from build123d import *

# Parameters (mm, degrees)
F0_W     = 8.3429142833
F0_H     = 111.0566146672
F1_DEPTH = 76.2
F0_W_2   = 108.8683158159
F0_H_2   = 0.4005401015
F2_DEPTH = 25.4
F3_SIZE  = 5.08
F4_DEPTH = 25.4


with BuildPart() as f1:
    # F0 (on Front) → F1 (new body)
    with BuildSketch(Plane.XZ):
        with Locations((-72.48769328, 5.1288474351)):
            Rectangle(F0_W, F0_H)
    extrude(amount=F1_DEPTH)



with BuildPart() as f1b:
    # F0 (on Front) → F1, piece 2 (new body)
    with BuildSketch(Plane.XZ):
        with Locations((-13.8820782304, -50.5997299492)):
            Rectangle(F0_W_2, F0_H_2)
    extrude(amount=F1_DEPTH)


with BuildPart() as f1_1:
    add(f1.part)
    # F2 (add): a face of the model
    f2_faces = [f1b.part.faces().sort_by_distance(p)[0] for p in [
        (-68.3162361383, -38.1, -50.5997299492),
    ]]

    add(f1b.part)  # F2 merges F1b
    extrude(f2_faces, amount=F2_DEPTH)

    # F3
    f3_edges = [f1_1.edges().sort_by_distance(p)[0] for p in [
        (-76.65915, -38.1, 60.657155),
        (-72.487693, 0, 60.657155),
    ]]
    chamfer(f3_edges, length=F3_SIZE)

    # F4 (add): a face of the model
    f4_faces = [f1_1.faces().sort_by_distance(p)[0] for p in [
        (-74.1483458239, -39.3554022989, 58.0879593664),
    ]]
    extrude(f4_faces, amount=F4_DEPTH)


solid = f1_1.part
Can you work these out from the model? Positions are in its coordinate system, mm. A direction names the side the tool comes from. Coordinates: 2 decimals unless noted, no trailing zeros. Write each loop counter-clockwise with the first axis right and the second up, starting at its lowest first coordinate (ties: lowest second). Pieces come first, ordered by that corner, then holes. Notation, with made-up numbers: (-0.75, 32.25) -> (13.25, 32.25) arc R17 ccw to (13.25, 50.25) -> close; hole circle Ø1 at (68.25, 40). An arc over 180 degrees is marked (long way). Write item = value, one per line.
(1) Imagine slicing it at C-C (x = 28.5). Please give me the cut outline in (y, z).
Verdict:
outline = (-76.2, -50.8) -> (0, -50.8) -> (0, -50.4) -> (-76.2, -50.4) -> close
(2) If I drill on probe 1 along X at (y, z) = (-52, -27.5); probe 2 along Z at (x, y) = (-16.5, -33); probe 3 along X at (y, z) = (-54, 71), over which ranges is the centre line in solid material (lowest first)?
Verdict:
probe_1 = -76.66 to -68.32
probe_2 = -50.8 to -50.4
probe_3 = -92.08 to -81.92
(3) Imagine slicing it at B-B (z = 49). Please give me the cut outline in (x, y), and give its area (3 significant figures).
Verdict:
outline = (-76.66, -76.2) -> (-68.32, -76.2) -> (-68.32, 0) -> (-76.66, 0) -> close
area = 636 mm^2
(4) Imagine slicing it at A-A (y = -47.5). Please give me the cut outline in (x, z).
Verdict:
outline = (-94.62, 73.54) -> (-76.66, 55.58) -> (-76.66, -50.4) -> (-93.72, -50.4) -> (-93.72, -50.8) -> (40.55, -50.8) -> (40.55, -50.4) -> (-68.32, -50.4) -> (-68.32, 60.66) -> (-71.58, 60.66) -> (-89.54, 78.62) -> close
(5) Thinking about a two-plate mould opening in Z: for faces 1 (the face through (-68.316, -38, 4)), 2 (the face through (-76.659, -38, 2)), 3 (the face through (-26, -38, -50.8)), 4 (the face through (-82.938, -2.576, 67.007)), which applies, +Z half, -Z half, draft (parallel to the pull), parting line (faces both ways), or undercut?
Verdict:
face_1 = draft
face_2 = undercut
face_3 = -Z half
face_4 = +Z half
(6) For pin 1 (6 mm diameter, centred on y = -14, z = -22, fed in from -X); pin 2 (3.5 mm diameter, centred on x = -70, y = -46.5, fed in from +Z); pin 3 (1 mm diameter, centred on x = -40, y = -23, fed in from +Z), each with a flat end and sliding along its axis, tell me the tip position at first contact or that it passes through.
Verdict:
pin_1 = -76.66
pin_2 = 60.83
pin_3 = -50.4
(7) On a 3-axis mill with a long thin cutter (end or side, diameter ignored), from which of +Z, -Z, +X, -X, +Y, -Y can I reach the whole of each face in a straight line? I mean faces 5 (the face through (-71.619, -1.94, 57.517)), 6 (the face through (-85, -38, -50.399)), 7 (the face through (-71, 0, 2)), 8 (the face through (-70, -40, 60.657)), 9 (the face through (-92.12, -37.57, 76.04)). Say none if no direction works.
Verdict:
face_5 = +Z, +X, +Y
face_6 = -X, +Y, -Y
face_7 = +Z, -Z, +X, -X, +Y
face_8 = +Z, +X, +Y, -Y
face_9 = +Z, -X, +Y, -Y
